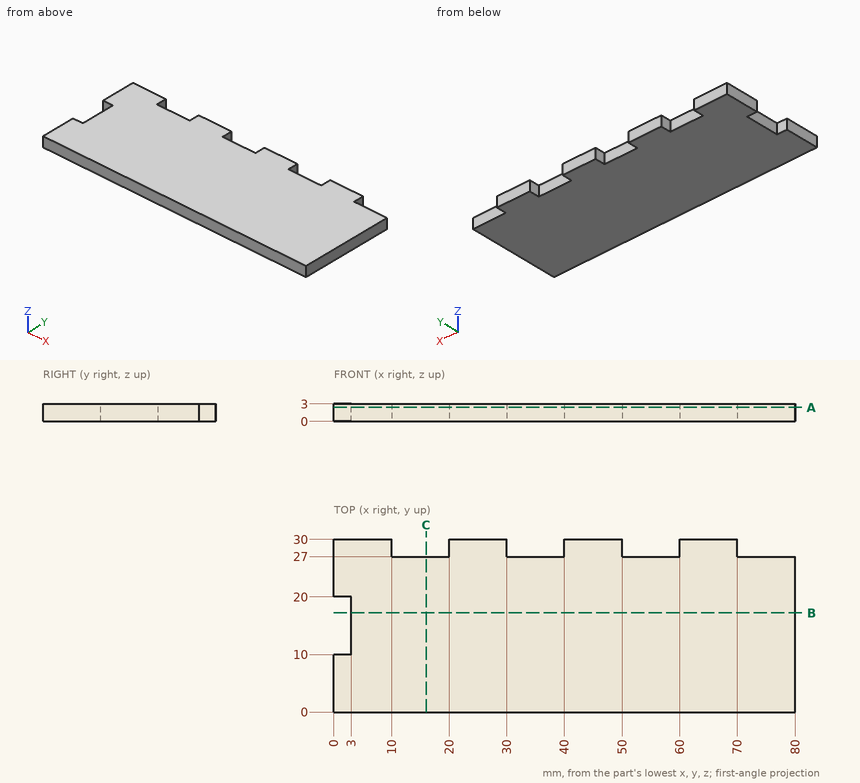
The figure shows three views and two pictorial views of one solid part (mm, origin at its lowest corner). Answer the questions. Give positions to 0.01 mm unless a question says otherwise; leave off trailing zeros. Order: outer loops, then holes, each group sorted by start corner. A loop starts at its lowest first (then second) coordinate and runs counter-clockwise, first axis right, second up. Notation, with made-up numbers: (79, 4) -> (104, 4) arc R13 cw to (104, 25) -> close; hole circle Ø6 at (30, 29.5). An arc over 180 degrees is marked (long way). Answer as a JSON object with one key per item and string values. Group by question number.
Item 1: The part is cut by section C-C on x = 16. Write down the section's boundary in (y, z).
Item 2: The part is cut by section B-B on y = 17.25. Write down the section's boundary in (x, z), and give its area (3 significant figures).
Item 3: The part is cut by section A-A on z = 2.4. Write down the section's boundary in (x, y).
Item 4: Consider L1, parallel to Y at x = 57, z = 0.75; L2, parallel to X at y = 11.5, z = 0.45. Determine where each line is inside the solid, lowest interval first. Write a range as from..to.
Item 5: Flat-ended cylindrical pins translate along their axes: pin 1 (0.9 mm diameter, centred on x = 73, z = 2, fed in from +Y); pin 2 (0.9 mm diameter, centred on y = 13, z = 1.5, fed in from -X); pin 3 (0.9 mm diameter, centred on y = 29, z = 2, fed in from +X). Find the tip coordinate at first contact, or state that the pin passes through.
Result set:
{
 "1": {"outline": "(0, 0) -> (27, 0) -> (27, 3) -> (0, 3) -> close"},
 "2": {"outline": "(3, 0) -> (80, 0) -> (80, 3) -> (3, 3) -> close", "area": "231 mm²"},
 "3": {"outline": "(0, 0) -> (80, 0) -> (80, 27) -> (70, 27) -> (70, 30) -> (60, 30) -> (60, 27) -> (50, 27) -> (50, 30) -> (40, 30) -> (40, 27) -> (30, 27) -> (30, 30) -> (20, 30) -> (20, 27) -> (10, 27) -> (10, 30) -> (0, 30) -> (0, 20) -> (3, 20) -> (3, 10) -> (0, 10) -> close"},
 "4": {"L1": "0..27", "L2": "3..80"},
 "5": {"pin 1": "y = 27", "pin 2": "x = 3", "pin 3": "x = 70"}
}
